```python
from build123d import *
from build123d.topology import SkipClean

# Parameters (mm, degrees)
BASE_EXTRUDE_DEPTH  = 9.525
SKETCH2_W           = 101.6
SKETCH2_H           = 12.7
BOSS_EXTRUDE1_DEPTH = 53.975
SKETCH3_R           = 25.4
BOSS_EXTRUDE2_DEPTH = 31.75
SKETCH4_R           = 14.2875
CUT_EXTRUDE1_DEPTH  = 121.858701073
RIB1_START          = -5
RIB1_DEPTH          = 10


# Read off the part's stored shape, not the designer's step: Rib1
with BuildPart() as part:
    # Sketch1 → Base-Extrude (new body)
    with BuildSketch(Plane.XY):
        with BuildLine():
            Line((-50.8, -101.6), (50.8, -101.6))
            Line((50.8, -101.6), (50.8, -88.9))
            Line((50.8, -88.9), (24.490190652, 6.737251801))
            ThreePointArc((24.490190652, 6.737251801), (0, 25.4), (-24.490190652, 6.737251801))
            Line((-24.490190652, 6.737251801), (-50.8, -88.9))
            Line((-50.8, -88.9), (-50.8, -101.6))
        make_face()
    extrude(amount=BASE_EXTRUDE_DEPTH)

    # Sketch2 → Boss-Extrude1 (add)
    with BuildSketch(Plane.XY.offset(9.525)):
        with Locations((0, -95.25)):
            Rectangle(SKETCH2_W, SKETCH2_H)
    extrude(amount=BOSS_EXTRUDE1_DEPTH)

    # Sketch3 → Boss-Extrude2 (add)
    with BuildSketch(Plane.XY.offset(9.525)):
        with Locations(Location((0, 0, 0), (0, 0, 164.618421377))):
            Circle(SKETCH3_R)
    extrude(amount=BOSS_EXTRUDE2_DEPTH)

    # Sketch4 → Cut-Extrude1 (cut, through all)
    with BuildSketch(Plane.XY.offset(41.275)):
        Circle(SKETCH4_R)
    extrude(amount=-CUT_EXTRUDE1_DEPTH, mode=Mode.SUBTRACT)

    # Rib1 outline → Rib1 (add)
    with SkipClean():  # the faces are left unmerged after this step: merging them gives an invalid solid
        with BuildSketch(Plane(origin=(0, 0, 0), x_dir=(0, 0, -1), z_dir=(1, 0, 0)).offset(RIB1_START)):
            Polygon((-41.101054153, -24.903011866), (-63.5, -88.9), (-9.525, -88.9), (-9.525, -23), (-40.435, -23), align=None)
        extrude(amount=RIB1_DEPTH)


solid = part.part
```
Source: CAD feature listing. Evaluate the final solid. Frame: model axes, mm. A direction names the side the tool comes from. Coordinates: 2 decimals unless noted, no trailing zeros. Loops run counter-clockwise (first coordinate to the right, second up) from the corner with the lowest first, then second, coordinate; pieces in that order, holes last. Notation, with made-up numbers: (13.5, -15) - (61.5, -15) arc R16 cw to (61.5, 15) - close; hole circle Ø11 at (-2, 89). An arc over 180 degrees is marked (long way). Answer as CSV lines item,"result".
1. Contact query for flat-ended pins moving along their axis: pin 1 (23 mm diameter, centred on x = -28, y = -21, fed in from +Z) (3 decimals); pin 2 (2 mm diameter, centred on x = -38.5, z = 33.5, fed in from +Y); pin 3 (23 mm diameter, centred on x = 17.5, z = 23.5, fed in from +Y). Output: stop coordinate, or through.
Established:
pin 1,"stops at z = 41.275"
pin 2,"stops at y = -88.9"
pin 3,"stops at y = 24.68"
2. Section A-A (z = 7). Return loops of the section in (x, y) (1 decimal).
Established:
outline,"(-50.8, -101.6) - (50.8, -101.6) - (50.8, -88.9) - (24.5, 6.7) arc R25.4 ccw to (-24.5, 6.7) - (-50.8, -88.9) - close; hole circle Ø28.6 at (0, 0)"
3. Section B-B (y = 0). Return loops of the section in (x, z) (1 decimal), then the cut area to 3 significant figures.
Established:
outline,"(-26.3, 0) - (-14.3, 0) - (-14.3, 41.3) - (-25.4, 41.3) - (-25.4, 9.5) - (-26.3, 9.5) - close; (14.3, 0) - (26.3, 0) - (26.3, 9.5) - (25.4, 9.5) - (25.4, 41.3) - (14.3, 41.3) - close"
area,"935 mm2"
4. Mould query, pull axis X, two halves, no side actions, for faces 4 (the cylindrical face through (-14.274, 0.628, 20.926)), 5 (the flat face through (-0.07, -56.454, 52.144)), 6 (the flat face through (-5, -56, 31)). Classes: released by +X, released by -X, zero draft, split by the parting line, or undercut.
Established:
face 4,"undercut"
face 5,"zero draft"
face 6,"released by -X"
5. Reachability of faces 1 (the flat face through (-23, -51, 9.525)), 2 (the flat face through (-8, 13, 41.275)), 3 (the flat face through (22, -51, 9.525)) from +Z, -Z, +X, -X, +Y, -Y: full face, straight path, thin tool, end or side. Return the list, or none.
Established:
face 1,"+Z, -X"
face 2,"+Z, +X, -X, +Y"
face 3,"+Z, +X"
6. Section D-D (y = -45). Return loops of the section in (x, z) (3 decimals), then the cut area to 3 significant figures.
Established:
outline,"(-38.723, 0) - (38.723, 0) - (38.723, 9.525) - (5, 9.525) - (5, 48.135) - (-5, 48.135) - (-5, 9.525) - (-38.723, 9.525) - close"
area,"1,120 mm2"
7. Section C-C (x = -21). Return loops of the section in (y, z) (3 decimals), then the cut area to 3 significant figures.
Established:
outline,"(-101.6, 0) - (14.288, 0) - (14.288, 41.275) - (-14.288, 41.275) - (-14.288, 9.525) - (-88.9, 9.525) - (-88.9, 63.5) - (-101.6, 63.5) - close"
area,"2,700 mm2"
8. Ray query, line 1 (Y direction, x = 0, z = 13); line 2 (Y direction, x = -39, z = 34); line 3 (Y direction, x = 10, z = 10). Return the intervals inside material, ascending.
Established:
line 1,"y = -101.6 to -14.29, 14.29 to 25.4"
line 2,"y = -101.6 to -88.9"
line 3,"y = -101.6 to -88.9, -23.35 to -10.2, 10.2 to 23.35"
